```python
from build123d import *

# Parameters (mm, degrees)
BOSS_EXTRUDE1_DEPTH                             = 6
CSK_FOR_M4_FLAT_HEAD_MACHINE_SCREW1_D           = 4.5
CSK_FOR_M4_FLAT_HEAD_MACHINE_SCREW1_CSINK_D     = 9.4
CSK_FOR_M4_FLAT_HEAD_MACHINE_SCREW1_CSINK_ANGLE = 90
CUT_EXTRUDE1_DEPTH                              = 88.740146645
CUT_EXTRUDE1_DEPTH_BACK                         = 88.740146645
SKETCH3_R                                       = 2
CUT_EXTRUDE3_START                              = -3
CUT_EXTRUDE3_DEPTH                              = 10


with BuildPart() as part:
    # Sketch2 → Boss-Extrude1 (new body)
    with BuildSketch(Plane(origin=(0, 0, 0), x_dir=(1, 0, 0), z_dir=(0, 1, 0))):
        Polygon((-6, 64.663230149), (-59, -27.135462652), (-53, -37.527767497), (53, -37.527767497), (59, -27.135462652), (6, 64.663230149), align=None)
    extrude(amount=BOSS_EXTRUDE1_DEPTH)

    # CSK for M4 Flat Head Machine Screw1 (through all)
    with Locations(Plane(origin=(0, 6, 0), x_dir=(1, 0, 0), z_dir=(0, 1, 0))):
        with Locations((0, 0)):
            CounterSinkHole(CSK_FOR_M4_FLAT_HEAD_MACHINE_SCREW1_D / 2, CSK_FOR_M4_FLAT_HEAD_MACHINE_SCREW1_CSINK_D / 2, counter_sink_angle=CSK_FOR_M4_FLAT_HEAD_MACHINE_SCREW1_CSINK_ANGLE)

    # Sketch3 → Cut-Extrude1 (cut, two sides: drawn at the far end of the back side and taken through both)
    with BuildSketch(Plane(origin=(0, 6, 0), x_dir=(1, 0, 0), z_dir=(0, 1, 0)).offset(-CUT_EXTRUDE1_DEPTH_BACK)):
        with Locations(Location((-47.372740925, -26.780019623, 0), (0, 0, 270))):
            Circle(SKETCH3_R)
        with Locations(Location((0.494193155, 54.416006899, 0), (0, 0, 270))):
            Circle(SKETCH3_R)
        with Locations(Location((46.87854777, -27.635987277, 0), (0, 0, 270))):
            Circle(SKETCH3_R)
    extrude(amount=CUT_EXTRUDE1_DEPTH + CUT_EXTRUDE1_DEPTH_BACK, mode=Mode.SUBTRACT)

    # Sketch7 → Cut-Extrude3 (cut)
    with BuildSketch(Plane(origin=(0, 6, 0), x_dir=(1, 0, 0), z_dir=(0, 1, 0)).offset(CUT_EXTRUDE3_START)):
        Polygon((-43.775560598, -25.136509042), (-46.997472676, -22.843014787), (-50.594653003, -24.486525368), (-50.969921252, -28.423530203), (-47.748009174, -30.717024458), (-44.150828847, -29.073513878), align=None)
        Polygon((3.716105233, 52.122512644), (4.091373482, 56.05951748), (0.869461405, 58.353011735), (-2.727718922, 56.709501154), (-3.102987172, 52.772496319), (0.118924906, 50.479002064), align=None)
        Polygon((43.281367443, -29.279497857), (46.50327952, -31.572992112), (50.100459847, -29.929481531), (50.475728097, -25.992476696), (47.253816019, -23.698982441), (43.656635692, -25.342493022), align=None)
    extrude(amount=-CUT_EXTRUDE3_DEPTH, mode=Mode.SUBTRACT)


solid = part.part
```
Here's how the part is built. I have some questions about the finished solid (model axes, mm). A direction names the side the tool comes from. Give positions to 0.01 mm unless a question says otherwise; leave off trailing zeros. Order: outer loops, then holes, each group sorted by start corner. A loop starts at its lowest first (then second) coordinate and runs counter-clockwise, first axis right, second up. Notation, with made-up numbers: (64, 2.5) - (76, 2.5) arc R27 ccw to (76, 32.5) - close; hole circle Ø7 at (57, -39). An arc over 180 degrees is marked (long way). Answer as a JSON object with one key per item and string values. Group by question number.
Item 1: If we section it at A-A on y = 1.25: Please give me the cut outline in (x, z).
Item 2: If we section it at D-D on z = -26.5: Please give me the cut outline in (x, y).
Item 3: Which directions (+Z, -Z, +X, -X, +Y, -Y) give clear straight access to the entire face, cutting with the end or side of a thin tool? Please do faces 1 (the flat face through (-43.966, 1.521, 27.133)), 2 (the cylindrical face through (0.29, 1.75, -2.23)).
Item 4: Please list where these lines run through material, in increasing order: probe 1 along Z at (x, y) = (-1, 1.35); probe 2 along X at (y, z) = (2.6, -55); probe 3 along Z at (x, y) = (-48.5, 1.95).
Item 5: For P1, Ø3, axis at y = 3, z = -26.5, coming from the -X side; P2, Ø2, axis at x = -1, z = -56, coming from the -Y side, each with a flat end and sliding along its axis, tell me the tip position at first contact or that it passes through.
Item 6: If we section it at B-B on z = 0: Please give me the cut outline in (x, y).
Item 7: If we section it at C-C on x = 30: Please give me the cut outline in (y, z).
Item 8: If we mould it in two halves opening along X, with no side actions, what happens to faces 3 (the flat face through (-56.04, 2.96, 32.26)), 4 (the flat face through (-45.36, 1.52, 24.01)), 5 (the flat face through (55.96, 2.96, 32.4)), 6 (the flat face through (-1, 6, 8))? For each: pulls with the +X half, pulls with the -X half, needs draft (parallel to the pull), parting line crosses it, or undercut.
Result set:
{
 "1": {"outline": "(-59, 27.14) - (-6, -64.66) - (6, -64.66) - (59, 27.14) - (53, 37.53) - (-53, 37.53) - close; hole (-50.97, 28.42) - (-50.59, 24.49) - (-47, 22.84) - (-43.78, 25.14) - (-44.15, 29.07) - (-47.75, 30.72) - close; hole (-3.1, -52.77) - (-2.73, -56.71) - (0.87, -58.35) - (4.09, -56.06) - (3.72, -52.12) - (0.12, -50.48) - close; hole circle Ø4.5 at (0, 0); hole (43.28, 29.28) - (43.66, 25.34) - (47.25, 23.7) - (50.48, 25.99) - (50.1, 29.93) - (46.5, 31.57) - close"},
 "2": {"outline": "(-28.03, 0) - (28.03, 0) - (28.03, 6) - (-28.03, 6) - close"},
 "3": {"face 1": "-Y", "face 2": "+Y, -Y"},
 "4": {"probe 1": "-64.66 to -57.5, -51.28 to -2.02, 2.02 to 37.53", "probe 2": "-11.58 to -2.89, 3.99 to 11.58", "probe 3": "8.95 to 23.53, 30.18 to 37.53"},
 "5": {"P1": "x = -28.9", "P2": "y = 3"},
 "6": {"outline": "(-43.33, 0) - (-2.25, 0) - (-2.25, 3.55) - (-4.7, 6) - (-43.33, 6) - close; (2.25, 0) - (43.33, 0) - (43.33, 6) - (4.7, 6) - (2.25, 3.55) - close"},
 "7": {"outline": "(0, -23.09) - (6, -23.09) - (6, 37.53) - (0, 37.53) - close"},
 "8": {"face 3": "pulls with the -X half", "face 4": "undercut", "face 5": "pulls with the +X half", "face 6": "needs draft"}
}
